Geometry: see drawing. Coordinates: mm, zero at the bounding-box minimum. A direction names the side the tool comes from. Coordinates: 2 decimals unless noted, no trailing zeros. Write each loop counter-clockwise with the first axis right and the second up, starting at its lowest first coordinate (ties: lowest second). Pieces come first, ordered by that corner, then holes. Notation, with made-up numbers: (23, -27) -> (49, -27) arc R20 ccw to (49, -20) -> close; hole circle Ø1 at (9.25, -30.5). An arc over 180 degrees is marked (long way). Use one line per item in the form item = value. Start each with the question number.
(1) Ray query, line 1 along X through (y, z) = (55.75, 25.4); line 2 along X through (y, z) = (31, 31) (1 decimal); line 3 along Y through (x, z) = (43.5, 18.5). Return the intervals inside material, ascending.
(2) Pull-direction query (Y, two-part tool) for the marked faces 3, 4 and 5; classes: released by +Y, released by -Y, zero draft, split by the parting line, or undercut.
(3) First-contact query: pin 1 (17 mm diameter, centred on x = 207.95, y = 31.75, fed in from +Z). Flat tip, straight axial feed; report the tip coordinate or a pass-through.
(4) Cut plane C-C on y = 6. Return the cut outline in (x, z), plus the area to 4 significant figures.
(5) Cut plane A-A on z = 25.4. State how many separate pieces and enclosed holes the cut face has, plus the area to 3 significant figures.
(6) Set-up query: the marked faces 1 and 2. Return all of +Z, -Z, +X, -X, +Y, -Y with unobstructed straight access to the full face (end or side cutting, diameter ignored); none if empty.
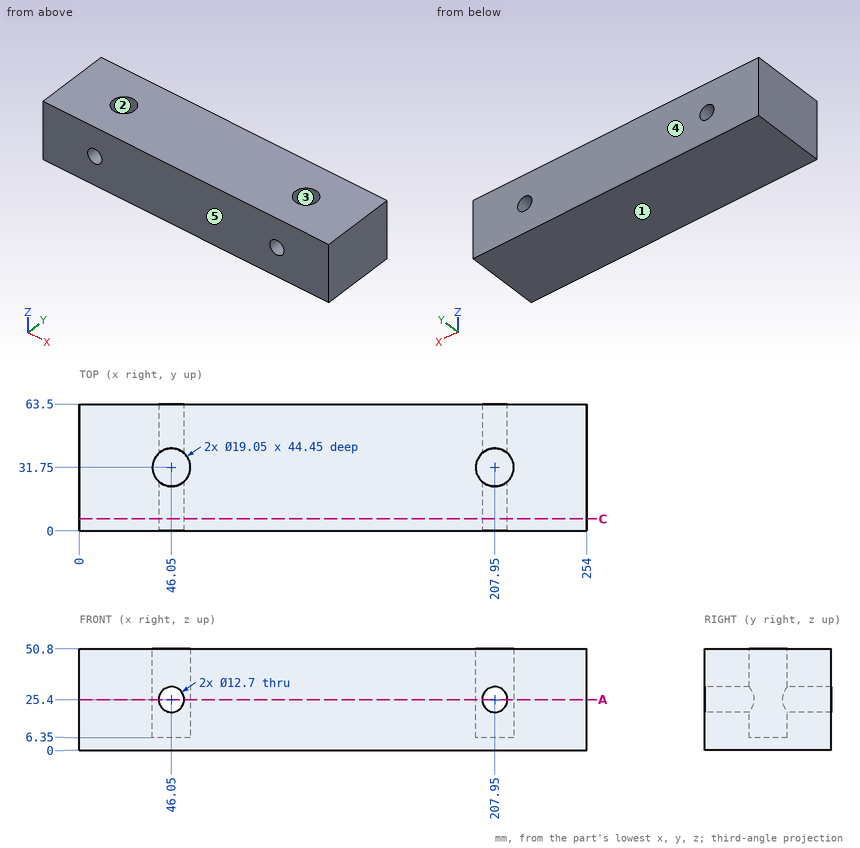
Values:
q1.line_1 = 0 to 39.7, 52.4 to 201.6, 214.3 to 254
q1.line_2 = 0 to 36.6, 55.5 to 198.5, 217.4 to 254
q1.line_3 = 0 to 22.57, 40.93 to 63.5
q2.face_3 = undercut
q2.face_4 = released by +Y
q2.face_5 = released by -Y
q3.pin_1 = 6.35
q4.outline = (0, 0) -> (254, 0) -> (254, 50.8) -> (0, 50.8) -> close; hole circle Ø12.7 at (46.05, 25.4); hole circle Ø12.7 at (207.95, 25.4)
q4.area = 12,650 mm2
q5.separate_pieces = 3
q5.enclosed_holes = 0
q5.area = 14,400 mm2
q6.face_1 = -Z, +X, -X, +Y, -Y
q6.face_2 = +Z
